```python
from build123d import *

# Parameters (mm, degrees)
F0_W     = 101
F0_H     = 19
F1_DEPTH = 5
F3_D     = 6
F5_D     = 10
F7_D     = 5


with BuildPart() as f1:
    # F0 (on Top) → F1 (new body)
    with BuildSketch(Plane.XY):
        Rectangle(F0_W, F0_H)
    extrude(amount=F1_DEPTH)

    # F3 (through all)
    with Locations(Plane.XY.offset(5)):
        with Locations((25.5, 0), (45.5, 0)):
            Hole(F3_D / 2)

    # F5 (through all)
    with Locations(Plane.XY.offset(5)):
        with Locations((-41.5, 0)):
            Hole(F5_D / 2)

    # F7 (through all)
    with Locations(Plane.XY.offset(5)):
        with Locations((-30, 4), (-20, 4), (-10, 4), (0, 4), (0, -4), (-10, -4), (-20, -4), (-30, -4)):
            Hole(F7_D / 2)


solid = f1.part
```
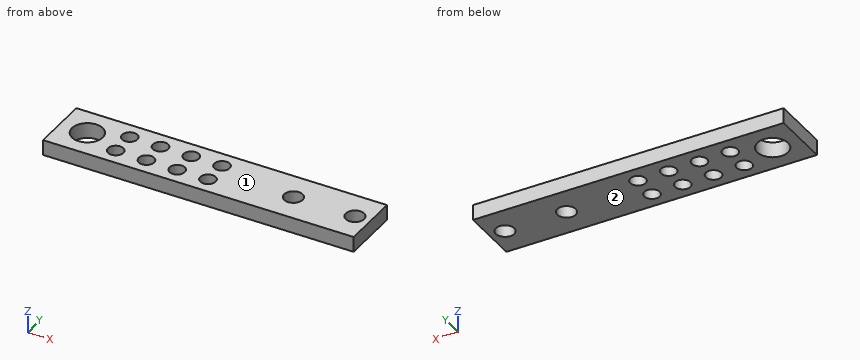
Part model, mm, in its own coordinate system. Face numbers are marked on the shaded views. Coordinates: 2 decimals unless noted, no trailing zeros. Write each loop counter-clockwise with the first axis right and the second up, starting at its lowest first coordinate (ties: lowest second). Pieces come first, ordered by that corner, then holes.
Item 1: Slice it at B-B (y = 4). Write the cut outline in (x, z).
Item 2: Mould opens along Z. For the marked faces 1 and 2 say: released by +Z, released by -Z, zero draft, split by the parting line, or undercut.
Item 3: Probe line 1 (Y direction, x = -10, z = 3.85); line 2 (X direction, y = -0.25, z = 3.1); line 3 (Y direction, x = 45.5, z = 1.75). List the from-to ranges inside material, lowest first.
Item 4: Slice it at A-A (x = -30). Write the cut outline in (y, z), and give its area (3 significant figures).
Item 5: Slice it at D-D (z = 2.4). Count the separate pieces of the cut face and the enclosed holes in it, and give its area (3 significant figures).
Item 6: Slice it at C-C (x = -41.5). Write the cut outline in (y, z).
Results found:
1. outline: (-50.5, 0) - (-44.5, 0) - (-44.5, 5) - (-50.5, 5) - close; (-38.5, 0) - (-32.5, 0) - (-32.5, 5) - (-38.5, 5) - close; (-27.5, 0) - (-22.5, 0) - (-22.5, 5) - (-27.5, 5) - close; (-17.5, 0) - (-12.5, 0) - (-12.5, 5) - (-17.5, 5) - close; (-7.5, 0) - (-2.5, 0) - (-2.5, 5) - (-7.5, 5) - close; (2.5, 0) - (50.5, 0) - (50.5, 5) - (2.5, 5) - close
2. face 1: released by +Z
2. face 2: released by -Z
3. line 1: y = -9.5 to -6.5, -1.5 to 1.5, 6.5 to 9.5
3. line 2: x = -50.5 to -46.49, -36.51 to 22.51, 28.49 to 42.51, 48.49 to 50.5
3. line 3: y = -9.5 to -3, 3 to 9.5
4. outline: (-9.5, 0) - (-6.5, 0) - (-6.5, 5) - (-9.5, 5) - close; (-1.5, 0) - (1.5, 0) - (1.5, 5) - (-1.5, 5) - close; (6.5, 0) - (9.5, 0) - (9.5, 5) - (6.5, 5) - close
4. area: 45.0 mm2
5. separate pieces: 1
5. enclosed holes: 11
5. area: 1,630 mm2
6. outline: (-9.5, 0) - (-5, 0) - (-5, 5) - (-9.5, 5) - close; (5, 0) - (9.5, 0) - (9.5, 5) - (5, 5) - close
